Part print with two shaded views. Sizes in mm from the minimum x, y, z corner. Give positions to 0.01 mm unless a question says otherwise; leave off trailing zeros. Write each loop counter-clockwise with the first axis right and the second up, starting at its lowest first coordinate (ties: lowest second). Pieces come first, ordered by that corner, then holes.
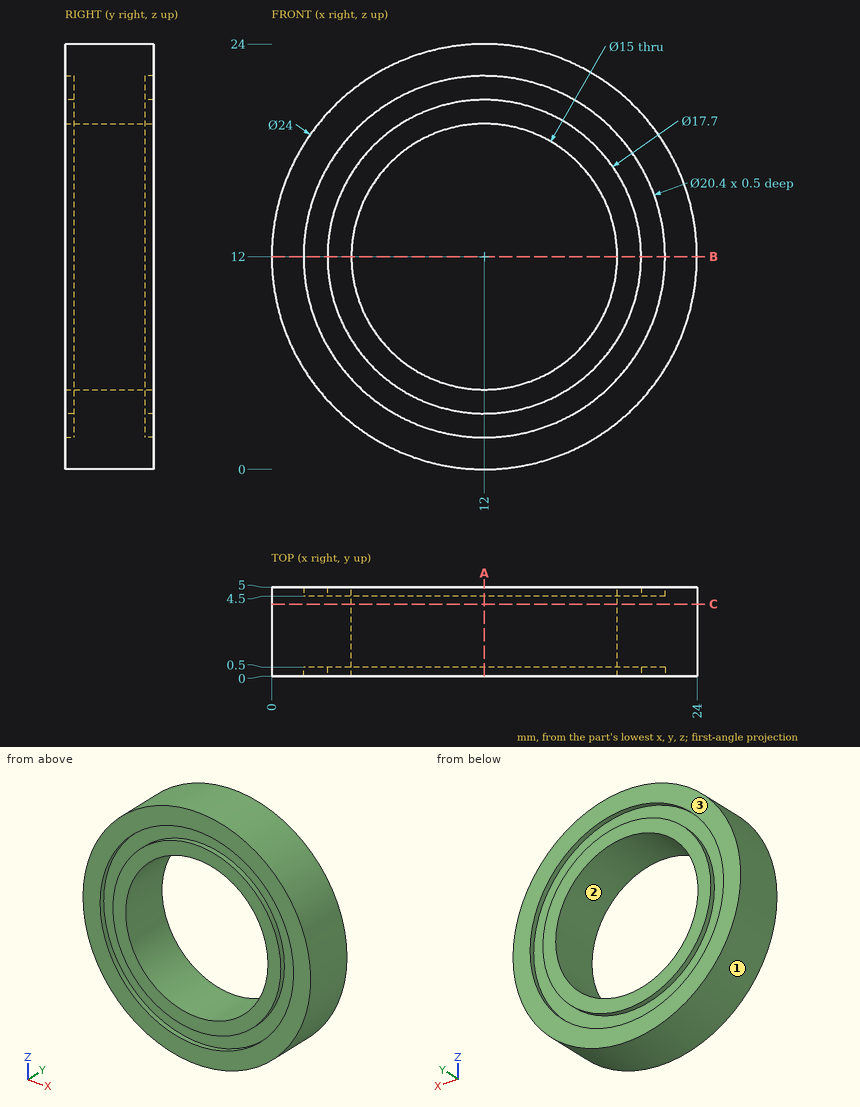
1) Saw through at A-A (x = 12). Write the cut outline in (y, z).
Check result:
outline: (0, 0) - (5, 0) - (5, 1.8) - (4.5, 1.8) - (4.5, 3.15) - (5, 3.15) - (5, 4.5) - (0, 4.5) - (0, 3.15) - (0.5, 3.15) - (0.5, 1.8) - (0, 1.8) - close; (0, 19.5) - (5, 19.5) - (5, 20.85) - (4.5, 20.85) - (4.5, 22.2) - (5, 22.2) - (5, 24) - (0, 24) - (0, 22.2) - (0.5, 22.2) - (0.5, 20.85) - (0, 20.85) - close
2) Saw through at B-B (z = 12). Write the cut outline in (x, y).
Check result:
outline: (0, 0) - (1.8, 0) - (1.8, 0.5) - (3.15, 0.5) - (3.15, 0) - (4.5, 0) - (4.5, 5) - (3.15, 5) - (3.15, 4.5) - (1.8, 4.5) - (1.8, 5) - (0, 5) - close; (19.5, 0) - (20.85, 0) - (20.85, 0.5) - (22.2, 0.5) - (22.2, 0) - (24, 0) - (24, 5) - (22.2, 5) - (22.2, 4.5) - (20.85, 4.5) - (20.85, 5) - (19.5, 5) - close
3) Saw through at C-C (y = 4.05). Write the cut outline in (x, z), and give its area (3 significant figures).
Check result:
outline: circle Ø24 at (12, 12); hole circle Ø15 at (12, 12)
area: 276 mm2
4) Mould opens along X. For the marked faces 1, 2 and 3 say: +X half, -X half, draft (parallel to the pull), parting line (faces both ways), or undercut.
Check result:
face 1: parting line
face 2: undercut
face 3: draft
5) Drill centre lines: L1, parallel to Z at x = 12, y = 4.6; L2, parallel to Z at x = 12, y = 3.4; L3, parallel to Z at x = 18.5, y = 1.9. Where is each one in solid material? Low to high.
Check result:
L1: z = 0 to 1.8, 3.15 to 4.5, 19.5 to 20.85, 22.2 to 24
L2: z = 0 to 4.5, 19.5 to 24
L3: z = 1.91 to 8.26, 15.74 to 22.09
6) Flat gauge pins, fed straight in: P1, Ø1, axis at y = 4.5, z = 15.5, coming from the -X side; P2, Ø3, axis at y = 3, z = 2.5, coming from the -X side. Where does each tip first touch, or does it go through?
Check result:
P1: stops at x = 0.38
P2: stops at x = 3.06
